Could you check a few things on this drawing? It's one solid part, dimensions in mm from its lowest x, y, z. A direction names the side the tool comes from. Give positions to 0.01 mm unless a question says otherwise; leave off trailing zeros. Loops run counter-clockwise (first coordinate to the right, second up) from the corner with the lowest first, then second, coordinate; pieces in that order, holes last. Notation, with made-up numbers: (8.25, -27) - (22.25, -27) arc R20 ccw to (22.25, -10) - close; hole circle Ø1 at (67, -25.75). An arc over 180 degrees is marked (long way). Write item = value, one per line.
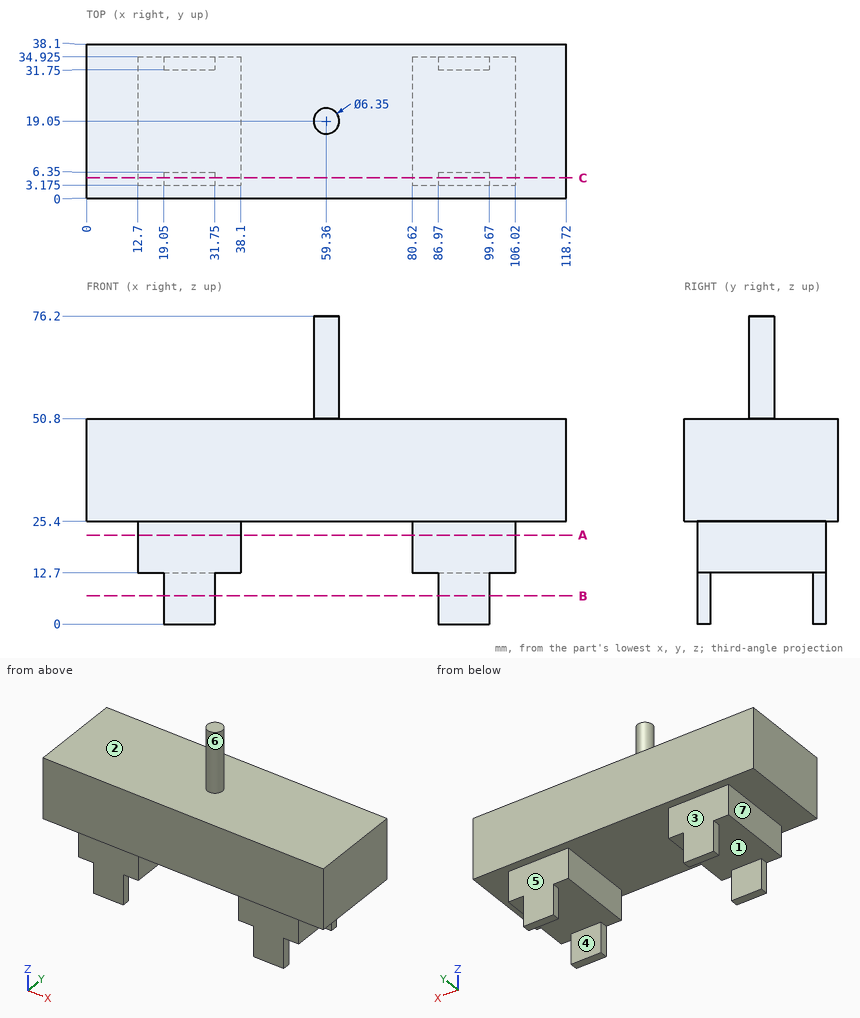
Q1. Which directions (+Z, -Z, +X, -X, +Y, -Y) give clear straight access to the entire face, cutting with the end or side of a thin tool? Please do the marked faces 4, 5, 6 and 7.
Output:
face_4 = -Z, +X, -X
face_5 = -Z, +X, -X, +Y
face_6 = +Z
face_7 = -Z, -X, +Y, -Y
Q2. Imagine slicing it at B-B, the plane z = 7. Give the number of separate pieces and of enclosed holes in the cut face, then the cut area to 3 significant figures.
Output:
separate_pieces = 4
enclosed_holes = 0
area = 161 mm2
Q3. Imagine slicing it at A-A, the plane z = 22. Write out the boundary of the cut face in (x, y) (1 decimal).
Output:
outline = (12.7, 3.2) - (38.1, 3.2) - (38.1, 34.9) - (12.7, 34.9) - close; (80.6, 3.2) - (106, 3.2) - (106, 34.9) - (80.6, 34.9) - close
Q4. We'd pull the mould along Y, two halves only. Please class the marked faces 1, 2 and 3: released by +Y, released by -Y, zero draft, split by the parting line, or undercut.
Output:
face_1 = undercut
face_2 = zero draft
face_3 = released by +Y
Q5. Imagine slicing it at C-C, the plane y = 5. Write out the boundary of the cut face in (x, z).
Output:
outline = (0, 25.4) - (12.7, 25.4) - (12.7, 12.7) - (19.05, 12.7) - (19.05, 0) - (31.75, 0) - (31.75, 12.7) - (38.1, 12.7) - (38.1, 25.4) - (80.62, 25.4) - (80.62, 12.7) - (86.97, 12.7) - (86.97, 0) - (99.67, 0) - (99.67, 12.7) - (106.02, 12.7) - (106.02, 25.4) - (118.72, 25.4) - (118.72, 50.8) - (0, 50.8) - close
Q6. I need wall thicknesses on L1, parallel to X at y = 17.5, z = 13; L2, parallel to Z at x = 51, y = 4.5; L3, parallel to Z at x = 18, y = 5. Which ranges of each line are inside material? Lowest first, please.
Output:
L1 = 12.7 to 38.1, 80.62 to 106.02
L2 = 25.4 to 50.8
L3 = 12.7 to 50.8
Q7. For pin 1 (4 mm diameter, centred on x = 104.5, z = 12.5, fed in from +Y) (3 decimals); pin 2 (14 mm diameter, centred on y = 19.5, z = 16.5, fed in from +X); pin 3 (1 mm diameter, centred on y = 5, z = 3.5, fed in from -X), each with a flat end and sliding along its axis, tell me the tip position at first contact or that it passes through.
Output:
pin_1 = 34.925
pin_2 = 106.02
pin_3 = 19.05
